Part model, mm, in its own coordinate system. A direction names the side the tool comes from. Coordinates: 2 decimals unless noted, no trailing zeros. Write each loop counter-clockwise with the first axis right and the second up, starting at its lowest first coordinate (ties: lowest second). Pieces come first, ordered by that corner, then holes. Notation, with made-up numbers: (-21.75, -0.75) - (35.25, -0.75) arc R35 ccw to (35.25, 34.25) - close; hole circle Ø2 at (-23, -39). An arc over 180 degrees is marked (long way). Use a Markdown table: item, result.
```python
from build123d import *

# Parameters (mm, degrees)
BOSS_EXTRUDE1_DEPTH = 1.6
SKETCH2_R           = 1
BOSS_EXTRUDE2_DEPTH = 9
FILLET1_R           = 2


with BuildPart() as part:
    # Sketch1 → Boss-Extrude1 (new body)
    with BuildSketch(Plane.XY):
        with BuildLine():
            Line((65.63056034, 41.616019999), (27.245760636, 41.591406461))
            Line((27.245760636, 41.591406461), (27.245760636, 22.351411618))
            Line((27.245760636, 22.351411618), (32.827326689, 22.351411618))
            Line((32.827326689, 22.351411618), (32.827326689, 3.745377262))
            Line((32.827326689, 3.745377262), (42.468635401, 3.745377262))
            Line((42.468635401, 3.745377262), (42.468635401, -13.000053658))
            Line((42.468635401, -13.000053658), (67.226484424, -13.000053658))
            Line((67.226484424, -13.000053658), (68.632483949, -8.295222112))
            Line((68.632483949, -8.295222112), (68.632483949, 38.616020588))
            ThreePointArc((68.632483949, 38.616020588), (67.753124087, 40.738020931), (65.63056034, 41.616019999))
        make_face()
    extrude(amount=BOSS_EXTRUDE1_DEPTH)

    # Sketch2 → Boss-Extrude2 (add)
    with BuildSketch(Plane(origin=(0, 0, 0), x_dir=(-1, 0, 0), z_dir=(0, 0, -1))):
        with Locations(Location((-30.536864632, 26.322094416, 0), (0, 0, 180))):
            Circle(SKETCH2_R)
        with Locations(Location((-45.827551279, -10.739617505, 0), (0, 0, 180))):
            Circle(SKETCH2_R)
        with Locations(Location((-61.773553069, -8.118356937, 0), (0, 0, 180))):
            Circle(SKETCH2_R)
        with Locations(Location((-64.977315986, 38.627456528, 0), (0, 0, 180))):
            Circle(SKETCH2_R)
    extrude(amount=BOSS_EXTRUDE2_DEPTH)

    # Fillet1
    fillet1_edges = [part.edges().sort_by_distance(p)[0] for p in [
        (68.632483949, -8.295222112, 0.8),
        (67.226484424, -13.000053658, 0.8),
        (42.468635401, -13.000053658, 0.8),
        (42.468635401, 3.745377262, 0.8),
        (32.827326689, 3.745377262, 0.8),
        (32.827326689, 22.351411618, 0.8),
        (27.245760636, 22.351411618, 0.8),
        (27.245760636, 41.591406461, 0.8),
    ]]
    fillet(fillet1_edges, radius=FILLET1_R)


solid = part.part
```
Item 1: Drill centre lines: probe 1 along Z at (x, y) = (62.5, -6); probe 2 along X at (y, z) = (39, 0.25); probe 3 along Y at (x, z) = (45, -3.75). Where is each one in solid material? Low to high.
From the geometry:
| item | result |
|---|---|
| probe 1 | 0 to 1.6 |
| probe 2 | 27.25 to 68.61 |
| probe 3 | -11.3 to -10.18 |
Item 2: Drop flat-ended pins along their axis: P1, Ø1.8, axis at x = 39, z = 0.5, coming from the -Y side; P2, Ø4, axis at x = 56, z = -3.5, coming from the +Y side; P3, Ø1.5, axis at x = 34.5, y = 8, coming from the -Z side; P4, Ø0.8, axis at y = 9.5, z = 1, coming from the -X side. Give the stop position or say it passes through.
From the geometry:
| item | result |
|---|---|
| P1 | y = 3.75 |
| P2 | through |
| P3 | z = 0 |
| P4 | x = 32.83 |
Item 3: Band-saw the part on B-B, the plane y = -2.5. Give the cut face in (x, z), then the cut area to 3 significant figures.
From the geometry:
| item | result |
|---|---|
| outline | (42.47, 0) - (68.63, 0) - (68.63, 1.6) - (42.47, 1.6) - close |
| area | 41.9 mm^2 |
Item 4: Band-saw the part on A-A, the plane x = 61.5. Give the cut face in (y, z).
From the geometry:
| item | result |
|---|---|
| outline | (-13, 0) - (-9.08, 0) - (-9.08, -9) - (-7.16, -9) - (-7.16, 0) - (41.61, 0) - (41.61, 1.6) - (-13, 1.6) - close |
Item 5: Band-saw the part on D-D, the plane y = 31. Give the cut face in (x, z), then the cut area to 3 significant figures.
From the geometry:
| item | result |
|---|---|
| outline | (27.25, 0) - (68.63, 0) - (68.63, 1.6) - (27.25, 1.6) - close |
| area | 66.2 mm^2 |
Item 6: Band-saw the part on C-C, the plane z = -6.5. Give the cut face in (x, y), then the cut area to 3 significant figures.
From the geometry:
| item | result |
|---|---|
| outline | circle Ø2 at (30.54, 26.32); circle Ø2 at (45.83, -10.74); circle Ø2 at (61.77, -8.12); circle Ø2 at (64.98, 38.63) |
| area | 12.6 mm^2 |
Item 7: Which spindle directions (+Z, -Z, +X, -X, +Y, -Y) get a long thin tool onto all of the face, cutting with end or side? Do faces 1 (the face through (68.095, -10.095, 0.789)), 2 (the face through (30, 22.351, 1)), 3 (the face through (64.2, 38, -4.4)). Say none if no direction does.
From the geometry:
| item | result |
|---|---|
| face 1 | +Z, -Z, +X, -Y |
| face 2 | +Z, -Z, -X, -Y |
| face 3 | -Z |
